Geometry: see drawing. Coordinates: mm, zero at the bounding-box minimum. Give positions to 0.01 mm unless a question says otherwise; leave off trailing zeros. One line per question, with ' | ' between items.
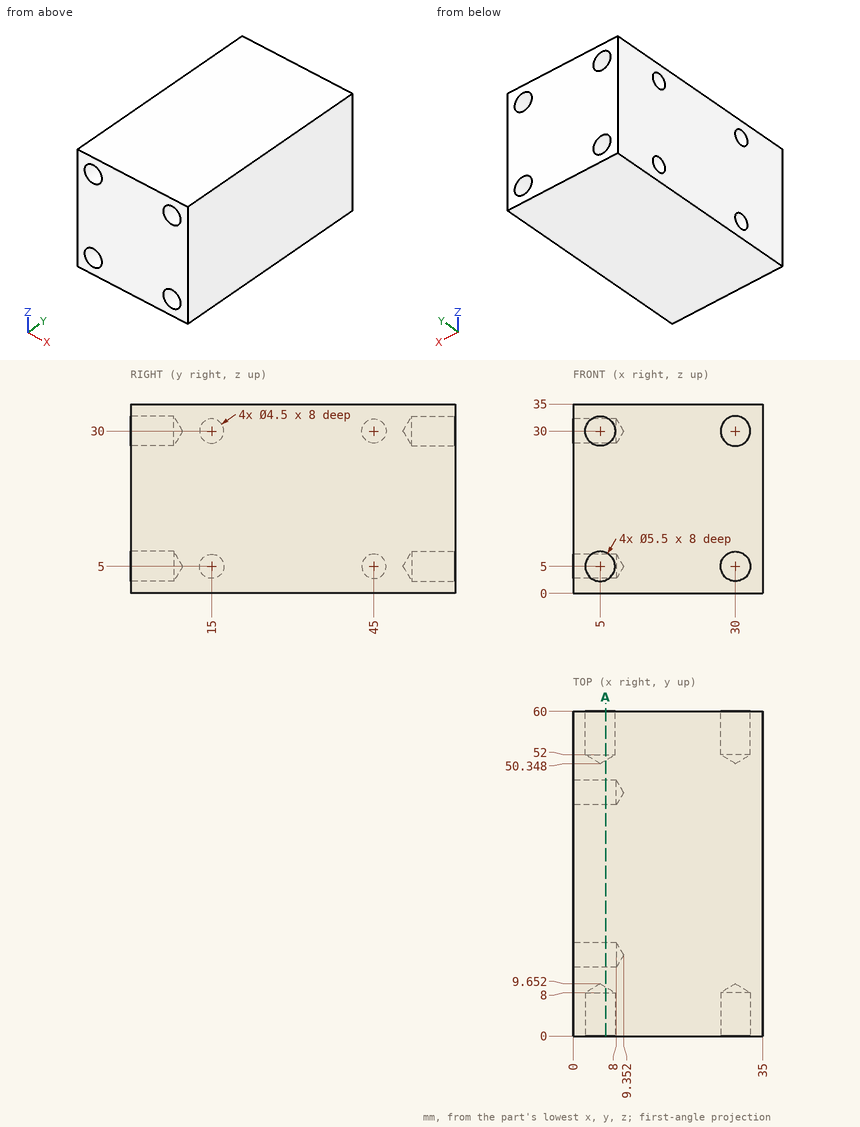
1. Section query A-A (x = 6). Count the separate pieces of the cut face and the enclosed holes in it, then the cut area to 3 significant figures.
Determined:
separate pieces: 1 | enclosed holes: 4 | area: 1,860 mm2
2. Pin query (flat end, axial travel): P1, Ø3.5, axis at x = 30, z = 30, coming from the +Y side; P2, Ø5, axis at x = 5, z = 5, coming from the +Y side; P3, Ø4.5, axis at x = 5, z = 5, coming from the +Y side. Return the tip coordinate at first contact, or that it passes through.
Determined:
P1: stops at y = 51.4 | P2: stops at y = 51.85 | P3: stops at y = 51.7
3. Ray query, line 1 along X through (y, z) = (55.75, 30); line 2 along Z through (x, y) = (3.25, 45); line 3 along Z through (x, y) = (6.5, 7.5) (1 decimal). Return the intervals inside material, ascending. Write a range as from..to.
Determined:
line 1: x = 0..2.25, 7.75..27.25, 32.75..35 | line 2: z = 0..2.75, 7.25..27.75, 32.25..35 | line 3: z = 0..2.7, 7.3..27.7, 32.3..35
